from build123d import *

# Parameters (mm, degrees)
ESQUISSE1_R             = 2.05
BOSS_EXTRU_2_DEPTH      = 17
ESQUISSE2_W             = 50
ESQUISSE2_H             = 2
BOSS_EXTRU_3_DEPTH      = 17
CONG_2_R                = 4
BOSS_EXTRU_4_DEPTH      = 1
CONG_3_R                = 0.4
CONG_4_R                = 2
ESQUISSE5_R             = 2.25
ENL_V_MAT_EXTRU_1_DEPTH = 2
CONG_5_R                = 5


with BuildPart() as part:
    # Esquisse1 → Boss.-Extru.2 (new body)
    with BuildSketch(Plane.XY):
        with BuildLine():
            Line((-8.75, 11.56233108), (-11.05949818, 11.56233108))
            ThreePointArc((-11.05949818, 11.56233108), (-13.925946075, 7.87832634), (-15.607142857, 3.523789414))
            ThreePointArc((-15.607142857, 3.523789414), (-21.5, 0), (-15.607142857, -3.523789414))
            ThreePointArc((-15.607142857, -3.523789414), (0, -16), (15.607142857, -3.523789414))
            ThreePointArc((15.607142857, -3.523789414), (21.5, 0), (15.607142857, 3.523789414))
            ThreePointArc((15.607142857, 3.523789414), (13.925946075, 7.87832634), (11.05949818, 11.56233108))
            Line((11.05949818, 11.56233108), (8.75, 11.56233108))
            ThreePointArc((8.75, 11.56233108), (0, -14.5), (-8.75, 11.56233108))
        make_face()
        with Locations((-17.5, 0)):
            Circle(ESQUISSE1_R, mode=Mode.SUBTRACT)
        with Locations((17.5, 0)):
            Circle(ESQUISSE1_R, mode=Mode.SUBTRACT)
    extrude(amount=BOSS_EXTRU_2_DEPTH)

    # Esquisse2 → Boss.-Extru.3 (add)
    with BuildSketch(Plane.XY.offset(17)):
        with Locations((0, -16)):
            Rectangle(ESQUISSE2_W, ESQUISSE2_H)
    extrude(amount=-BOSS_EXTRU_3_DEPTH)

    # Congé2
    cong_2_edges = [part.edges().sort_by_distance(p)[0] for p in [
        (5.567764363, -15, 8.5),
        (-5.567764363, -15, 8.5),
    ]]
    fillet(cong_2_edges, radius=CONG_2_R)

    # Esquisse4 → Boss.-Extru.4 (add)
    with BuildSketch(Plane(origin=(0, 0, 0), x_dir=(-1, 0, 0), z_dir=(0, 0, -1))):
        with BuildLine():
            Line((-1.414213562, 0), (-10.935743054, -9.521529492))
            ThreePointArc((-10.935743054, -9.521529492), (-10.600707524, -9.893179469), (-10.253048327, -10.253048327))
            ThreePointArc((-10.253048327, -10.253048327), (-9.893179469, -10.600707524), (-9.521529492, -10.935743054))
            Line((-9.521529492, -10.935743054), (0, -1.414213562))
            Line((0, -1.414213562), (9.521529492, -10.935743054))
            ThreePointArc((9.521529492, -10.935743054), (9.893179469, -10.600707524), (10.253048327, -10.253048327))
            ThreePointArc((10.253048327, -10.253048327), (10.600707524, -9.893179469), (10.935743054, -9.521529492))
            Line((10.935743054, -9.521529492), (1.414213562, 0))
            Line((1.414213562, 0), (10.935743054, 9.521529492))
            ThreePointArc((10.935743054, 9.521529492), (10.600707524, 9.893179469), (10.253048327, 10.253048327))
            ThreePointArc((10.253048327, 10.253048327), (9.893179469, 10.600707524), (9.521529492, 10.935743054))
            Line((9.521529492, 10.935743054), (0, 1.414213562))
            Line((0, 1.414213562), (-9.521529492, 10.935743054))
            ThreePointArc((-9.521529492, 10.935743054), (-10.253048327, 10.253048327), (-10.935743054, 9.521529492))
            Line((-10.935743054, 9.521529492), (-1.414213562, 0))
        make_face()
    extrude(amount=-BOSS_EXTRU_4_DEPTH)

    # Congé3
    cong_3_edges = [part.edges().sort_by_distance(p)[0] for p in [
        (-8.75, 11.56233108, 8.5),
        (8.75, 11.56233108, 8.5),
    ]]
    fillet(cong_3_edges, radius=CONG_3_R)

    # Congé4
    cong_4_edges = [part.edges().sort_by_distance(p)[0] for p in [
        (-10.935743054, -9.521529492, 0.5),
        (-9.521529492, -10.935743054, 0.5),
        (9.521529492, -10.935743054, 0.5),
        (10.935743054, -9.521529492, 0.5),
        (10.935743054, 9.521529492, 0.5),
        (-10.935743054, 9.521529492, 0.5),
    ]]
    fillet(cong_4_edges, radius=CONG_4_R)

    # Esquisse5 → Enlèv. mat.-Extru.1 (cut)
    with BuildSketch(Plane.XZ.offset(17)):
        with Locations(Location((-20, 8.5, 0), (0, 0, 270))):
            Circle(ESQUISSE5_R)
        with Locations(Location((20, 8.5, 0), (0, 0, 270))):
            Circle(ESQUISSE5_R)
    extrude(amount=-ENL_V_MAT_EXTRU_1_DEPTH, mode=Mode.SUBTRACT)

    # Congé5
    cong_5_edges = [part.edges().sort_by_distance(p)[0] for p in [
        (-25, -16, 17),
        (25, -16, 17),
        (-25, -16, 0),
        (25, -16, 0),
    ]]
    fillet(cong_5_edges, radius=CONG_5_R)


solid = part.part
Can you work these out from the model? Positions are in its coordinate system, mm. A direction names the side the tool comes from. Give positions to 0.01 mm unless a question says otherwise; leave off trailing zeros. Loops run counter-clockwise (first coordinate to the right, second up) from the corner with the lowest first, then second, coordinate; pieces in that order, holes last. Notation, with made-up numbers: (59, -0.75) -> (84, -0.75) arc R20 ccw to (84, 18.25) -> close; hole circle Ø10 at (-36, 45). An arc over 180 degrees is marked (long way). Use one line per item in the form item = value.
1) If we section it at A-A (z = 9): Please give me the cut outline in (x, y), plus the area to 3 significant figures.
Answers:
outline = (-25, -17) -> (-22.19, -17) -> (-22.19, -15) -> (-25, -15) -> close; (-17.81, -17) -> (17.81, -17) -> (17.81, -15) -> (16.7, -15) arc R4 cw to (13.36, -8.8) arc R16 ccw to (15.61, -3.52) arc R4 ccw (long way) to (15.61, 3.52) arc R16 ccw to (11.06, 11.56) -> (9.87, 11.56) arc R0.4 ccw to (9.6, 10.86) arc R14.5 cw (long way) to (-9.6, 10.86) arc R0.4 ccw to (-9.87, 11.56) -> (-11.06, 11.56) arc R16 ccw to (-15.61, 3.52) arc R4 ccw (long way) to (-15.61, -3.52) arc R16 ccw to (-13.36, -8.8) arc R4 cw to (-16.7, -15) -> (-17.81, -15) -> close; (22.19, -17) -> (25, -17) -> (25, -15) -> (22.19, -15) -> close; hole circle Ø4.1 at (-17.5, 0); hole circle Ø4.1 at (17.5, 0)
area = 272 mm²
2) If we section it at C-C (z = 14.5): Please give me the cut outline in (x, y).
Answers:
outline = (-24.33, -17) -> (24.33, -17) -> (24.33, -15) -> (16.7, -15) arc R4 cw to (13.36, -8.8) arc R16 ccw to (15.61, -3.52) arc R4 ccw (long way) to (15.61, 3.52) arc R16 ccw to (11.06, 11.56) -> (9.87, 11.56) arc R0.4 ccw to (9.6, 10.86) arc R14.5 cw (long way) to (-9.6, 10.86) arc R0.4 ccw to (-9.87, 11.56) -> (-11.06, 11.56) arc R16 ccw to (-15.61, 3.52) arc R4 ccw (long way) to (-15.61, -3.52) arc R16 ccw to (-13.36, -8.8) arc R4 cw to (-16.7, -15) -> (-24.33, -15) -> close; hole circle Ø4.1 at (-17.5, 0); hole circle Ø4.1 at (17.5, 0)
3) For faces 4 (the face through (5.296, -3.882, 0.493)), 5 (the face through (-4.833, 6.247, 0.493)), 6 (the face through (-23, -16, 16)), 7 (the face through (0, -1, 1)), which set-ups out of +Z, -Z, +X, -X, +Y, -Y let a thin tool reach every point of the face, with its end or its side?
Answers:
face_4 = +Z, -Z
face_5 = +Z, -Z, +Y
face_6 = +Z, -X, -Y
face_7 = +Z
4) We'd pull the mould along Z, two halves only. Please class faces 1 (the face through (-3.882, -5.296, 0.493)), 2 (the face through (-23, -16, 1)), 3 (the face through (17.804, -16.014, 8.988)): released by +Z, released by -Z, zero draft, split by the parting line, or undercut.
Answers:
face_1 = zero draft
face_2 = released by -Z
face_3 = undercut
5) If we section it at D-D (y = 5.25): Please give me the cut outline in (x, z), plus the area to 3 significant figures.
Answers:
outline = (-15.11, 0) -> (-13.52, 0) -> (-13.52, 17) -> (-15.11, 17) -> close; (-6.66, 0) -> (-3.84, 0) -> (-3.84, 1) -> (-6.66, 1) -> close; (3.84, 0) -> (6.66, 0) -> (6.66, 1) -> (3.84, 1) -> close; (13.52, 0) -> (15.11, 0) -> (15.11, 17) -> (13.52, 17) -> close
area = 60.0 mm²
6) If we section it at B-B (y = -4.75): Please give me the cut outline in (x, z), plus the area to 3 significant figures.
Answers:
outline = (-15.28, 0) -> (-13.7, 0) -> (-13.7, 17) -> (-15.28, 17) -> close; (-6.16, 0) -> (-3.34, 0) -> (-3.34, 1) -> (-6.16, 1) -> close; (3.34, 0) -> (6.16, 0) -> (6.16, 1) -> (3.34, 1) -> close; (13.7, 0) -> (15.28, 0) -> (15.28, 17) -> (13.7, 17) -> close
area = 59.3 mm²
7) I need wall thicknesses on line 1 along X through (y, z) = (-16.3, 8.5); line 2 along Y through (x, z) = (16.5, 3.75); line 3 along Y through (x, z) = (-17, 16.25). Which ranges of each line are inside material? Lowest first, please.
Answers:
line_1 = -25 to -22.25, -17.75 to 17.75, 22.25 to 25
line_2 = -17 to -14.99, -3.87 to -1.79, 1.79 to 3.87
line_3 = -17 to -15, -3.97 to -1.99, 1.99 to 3.97
8) Will these pins go through, and if not, where does the flat tip stop? pin 1 (3.5 mm diameter, centred on x = -20, z = 8.5, fed in from +Y); pin 2 (3.5 mm diameter, centred on x = -17.5, y = 0, fed in from +Z); pin 3 (6 mm diameter, centred on x = 20, z = 8.5, fed in from +Y); pin 4 (1.5 mm diameter, centred on y = 6.5, z = 6.5, fed in from -X).
Answers:
pin_1 = 3.93
pin_2 = through
pin_3 = 4
pin_4 = -14.93
